from build123d import *

# Parameters (mm, degrees)
SKETCH_W        = 56
SKETCH_H        = 120
PAD_DEPTH       = 4
SKETCH002_W     = 8
SKETCH002_H     = 8
PAD001_DEPTH    = 16
SKETCH003_R     = 1.4
POCKET_DEPTH    = 20
SKETCH004_R     = 1.8
POCKET001_DEPTH = 5
SKETCH006_W     = 7
SKETCH006_H     = 30
SKETCH006_W_2   = 9
PAD003_DEPTH    = 4
SKETCH007_W     = 4
SKETCH007_H     = 8
SKETCH007_W_2   = 8
SKETCH007_H_2   = 4
PAD004_DEPTH    = 6
SKETCH008_W     = 32
SKETCH008_H     = 50
POCKET002_DEPTH = 5


with BuildPart() as part:
    # Sketch → Pad (new body)
    with BuildSketch(Plane.XY):
        Rectangle(SKETCH_W, SKETCH_H)
    extrude(amount=PAD_DEPTH)

    # Sketch002 → Pad001 (join)
    with BuildSketch(Plane(origin=(0, 0, 0), x_dir=(1, 0, 0), z_dir=(0, 0, -1))):
        with Locations((24, 0)):
            Rectangle(SKETCH002_W, SKETCH002_H)
        with Locations((24, 56)):
            Rectangle(SKETCH002_W, SKETCH002_H)
        with Locations((-24, 56)):
            Rectangle(SKETCH002_W, SKETCH002_H)
        with Locations((-24, 0)):
            Rectangle(SKETCH002_W, SKETCH002_H)
    extrude(amount=PAD001_DEPTH)

    # Sketch003 (on Face26 of Pad001) → Pocket (cut)
    with BuildSketch(Plane(origin=(0, 0, -16), x_dir=(1, 0, 0), z_dir=(0, 0, -1))):
        with Locations((24.5, 57)):
            Circle(SKETCH003_R)
        with Locations((24.5, -1)):
            Circle(SKETCH003_R)
        with Locations((-24.5, -1)):
            Circle(SKETCH003_R)
        with Locations((-24.5, 57)):
            Circle(SKETCH003_R)
    extrude(amount=-POCKET_DEPTH, mode=Mode.SUBTRACT)

    # Sketch004 (on Face4 of Pocket) → Pocket001 (cut)
    with BuildSketch(Plane(origin=(0, 0, 0), x_dir=(1, 0, 0), z_dir=(0, 0, -1))):
        with Locations((0, -35)):
            Circle(SKETCH004_R)
        with Locations((0, -55)):
            Circle(SKETCH004_R)
        with Locations((15, -35)):
            Circle(SKETCH004_R)
        with Locations((15, -55)):
            Circle(SKETCH004_R)
        with Locations((-15, -35)):
            Circle(SKETCH004_R)
        with Locations((-15, -55)):
            Circle(SKETCH004_R)
        with Locations((15, 55)):
            Circle(SKETCH004_R)
        with Locations((0, 55)):
            Circle(SKETCH004_R)
        with Locations((-15, 55)):
            Circle(SKETCH004_R)
        with Locations((-15, 35)):
            Circle(SKETCH004_R)
        with Locations((0, 35)):
            Circle(SKETCH004_R)
        with Locations((15, 35)):
            Circle(SKETCH004_R)
    extrude(amount=-POCKET001_DEPTH, mode=Mode.SUBTRACT)

    # Sketch006 → Pad003 (join)
    with BuildSketch(Plane.XY):
        with Locations((-31.5, 21)):
            Rectangle(SKETCH006_W, SKETCH006_H)
        with Locations((32.5, 21)):
            Rectangle(SKETCH006_W_2, SKETCH006_H)
    extrude(amount=PAD003_DEPTH)

    # Sketch007 (on Face10 of Pad003) → Pad004 (join)
    with BuildSketch(Plane(origin=(0, 0, 0), x_dir=(1, 0, 0), z_dir=(0, 0, -1))):
        with Locations((35, -10)):
            Rectangle(SKETCH007_W, SKETCH007_H)
        with Locations((-33, -26)):
            Rectangle(SKETCH007_W, SKETCH007_H)
        with Locations((27, -34)):
            Rectangle(SKETCH007_W_2, SKETCH007_H_2)
        with Locations((-25, -34)):
            Rectangle(SKETCH007_W_2, SKETCH007_H_2)
    extrude(amount=PAD004_DEPTH)

    # Sketch008 (on Face4 of Pad004) → Pocket002 (cut)
    with BuildSketch(Plane(origin=(0, 0, 0), x_dir=(1, 0, 0), z_dir=(0, 0, -1))):
        Rectangle(SKETCH008_W, SKETCH008_H)
    extrude(amount=-POCKET002_DEPTH, mode=Mode.SUBTRACT)


solid = part.part
Read the model definition and answer for the solid it produces. Units are mm, in the model's axes. A direction names the side the tool comes from. Round coordinates to 2 decimals unless told otherwise and drop trailing zeros. Write each loop counter-clockwise with the first axis right and the second up, starting at its lowest first coordinate (ties: lowest second). Pieces come first, ordered by that corner, then holes.
1. Straight lines are drawn through the part: L1, parallel to Y at x = 24.5, z = -0.25; L2, parallel to X at y = -55, z = 2.4; L3, parallel to Y at x = -15, z = 2.8. For each, find the intervals that lie inside material, in ascending order.
2. Determine the mould class of faces 5 (the face through (0, -25, 2)), 6 (the face through (16, 0, 2)), 7 (the face through (24, -4, -8)), 8 (the face through (-29, 34, -3)) for opening direction X: pulls with the +X half, pulls with the -X half, needs draft (parallel to the pull), parting line crosses it, or undercut.
3. Given pin 1 Ø6.5 at (y, z) = (2, -12) entering from -X; pin 2 Ø1 at (x, z) = (20.5, -2.5) entering from +Y; pin 3 Ø2 at (y, z) = (35, -1.5) entering from -X; pin 4 Ø6 at (y, z) = (17.5, -4) entering from +X, each flat-ended and moving along its own axis, determine where each tip first touches the part or whether it passes through.
4. The part is cut by section C-C, the plane x = -10.5. Determine the outline of the cut face in (y, z).
5. The part is cut by section A-A, the plane z = -7.5. Determine the outline of the cut face in (x, y).
6. The part is cut by section D-D, the plane x = -24.5. Determine the outline of the cut face in (y, z).
7. Which of the six approach directions +Z, -Z, +X, -X, +Y, -Y give full straight-line access (tool end or side, diameter ignored) to faces 1 (the face through (-21, 34, -3)), 2 (the face through (33.4, 6, 0.2)), 3 (the face through (24, -52, -8)), 4 (the face through (35, 14, -3))?
8. The part is cut by section B-B, the plane y = 55. Determine the outline of the cut face in (x, z).
Values:
1. L1: y = -60 to -58.4, -55.6 to -52, -4 to -0.4, 2.4 to 4, 32 to 36
1. L2: x = -28 to -16.8, -13.2 to -1.8, 1.8 to 13.2, 16.8 to 28
1. L3: y = -60 to -56.8, -53.2 to -36.8, -33.2 to -25, 25 to 33.2, 36.8 to 53.2, 56.8 to 60
2. face 5: undercut
2. face 6: undercut
2. face 7: needs draft
2. face 8: pulls with the -X half
3. pin 1: stops at x = -28
3. pin 2: stops at y = 4
3. pin 3: stops at x = -29
3. pin 4: passes through
4. outline: (-60, 0) - (-25, 0) - (-25, 4) - (-60, 4) - close; (25, 0) - (60, 0) - (60, 4) - (25, 4) - close
5. outline: (-28, -60) - (-20, -60) - (-20, -52) - (-28, -52) - close; (-28, -4) - (-20, -4) - (-20, 4) - (-28, 4) - close; (20, -60) - (28, -60) - (28, -52) - (20, -52) - close; (20, -4) - (28, -4) - (28, 4) - (20, 4) - close; hole circle Ø2.8 at (-24.5, -57); hole circle Ø2.8 at (-24.5, 1); hole circle Ø2.8 at (24.5, -57); hole circle Ø2.8 at (24.5, 1)
6. outline: (-60, -16) - (-58.4, -16) - (-58.4, 4) - (-60, 4) - close; (-55.6, -16) - (-52, -16) - (-52, 0) - (-4, 0) - (-4, -16) - (-0.4, -16) - (-0.4, 4) - (-55.6, 4) - close; (2.4, -16) - (4, -16) - (4, 0) - (32, 0) - (32, -6) - (36, -6) - (36, 0) - (60, 0) - (60, 4) - (2.4, 4) - close
7. face 1: -Z, +Y
7. face 2: +Z, -Z, +X, -Y
7. face 3: -Z, +X, -X
7. face 4: -Z, +X, -X, +Y
8. outline: (-28, 0) - (-16.8, 0) - (-16.8, 4) - (-28, 4) - close; (-13.2, 0) - (-1.8, 0) - (-1.8, 4) - (-13.2, 4) - close; (1.8, 0) - (13.2, 0) - (13.2, 4) - (1.8, 4) - close; (16.8, 0) - (28, 0) - (28, 4) - (16.8, 4) - close
